The model under review builds one solid part; all positions refer to its coordinate system, in mm. Face numbers are marked on the shaded views. A direction names the side the tool comes from. Round coordinates to 2 decimals unless told otherwise and drop trailing zeros. Loops run counter-clockwise (first coordinate to the right, second up) from the corner with the lowest first, then second, coordinate; pieces in that order, holes last. Notation, with made-up numbers: (86, -11) -> (140, -11) arc R9 cw to (140, 2) -> close; hole circle Ø11 at (3, 86). An arc over 180 degrees is marked (long way). Use a Markdown table: item, result. Add a question column.
1) Insertion check: pin 1 (2 mm diameter, centred on y = -3.5, z = 5, fed in from +X); pin 2 (1.5 mm diameter, centred on x = 0.5, z = 12, fed in from -Y); pin 3 (2.5 mm diameter, centred on x = 0.5, y = 0, fed in from -Z). Each pin has a flat end and moves straight along its axis. Give the tip position at first contact, or say it passes through.
2) Wall thickness on probe 1 along Y at (x, z) = (0, 44); probe 2 along Z at (x, y) = (0.25, 3.25); probe 3 along Z at (x, y) = (-1.75, 0.5): over which ranges is each line inside the solid? List them lowest first.
3) For the marked faces 1 and 2, list the 3-axis set-ups (+Z, -Z, +X, -X, +Y, -Y) from which the entire face can be reached by the end or side of a thin tool; tool diameter is ignored.
4) Consider section A-A on y = 0. Give the boundary of the cut face in (x, z).
5) Consider section B-B on z = 41.5. Give the boundary of the cut face in (x, y).
from build123d import *

# Parameters (mm, degrees)
F0_R     = 4.73075
F1_DEPTH = 6.35
F2_R     = 3.0988
F3_DEPTH = 40.64
F5_DEPTH = 4.318
F6_SIZE  = 0.508


with BuildPart() as f1:
    # F0 (on Top) → F1 (new body)
    with BuildSketch(Plane.XY):
        Circle(F0_R)
    extrude(amount=F1_DEPTH)

    # F2 (on face) → F3 (join)
    with BuildSketch(Plane.XY.offset(6.35)):
        Circle(F2_R)
    extrude(amount=F3_DEPTH)

    # F4 (on face) → F5 (cut)
    with BuildSketch(Plane(origin=(0, 0, 0), x_dir=(1, 0, 0), z_dir=(0, 0, -1))):
        Polygon((2.38125, -1.374815), (2.38125, 1.374815), (0, 2.749631), (-2.38125, 1.374815), (-2.38125, -1.374815), (0, -2.749631), align=None)
    extrude(amount=-F5_DEPTH, mode=Mode.SUBTRACT)

    # F6
    f6_edges = [f1.edges().sort_by_distance(p)[0] for p in [
        (1.190625, 2.062223, 0),
        (2.38125, 0, 0),
        (1.190625, -2.062223, 0),
        (-1.190625, -2.062223, 0),
        (-2.38125, 0, 0),
        (-1.190625, 2.062223, 0),
        (-4.73075, 0, 0),
        (-4.73075, 0, 6.35),
        (-3.0988, 0, 46.99),
    ]]
    chamfer(f6_edges, length=F6_SIZE)


solid = f1.part
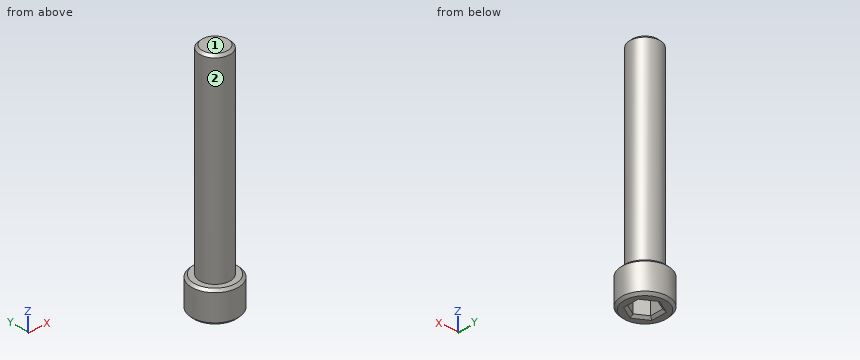
Result set:
| question | item | result |
|---|---|---|
| 1 | pin 1 | x = 4.02 |
| 1 | pin 2 | y = -3.1 |
| 1 | pin 3 | z = 4.32 |
| 2 | probe 1 | -3.1 to 3.1 |
| 2 | probe 2 | 0 to 6.35 |
| 2 | probe 3 | 4.32 to 46.99 |
| 3 | face 1 | +Z, +X, -X, +Y, -Y |
| 3 | face 2 | +Z |
| 4 | outline | (-4.73, 0.51) -> (-4.22, 0) -> (-2.89, 0) -> (-2.38, 0.51) -> (-2.38, 4.32) -> (2.38, 4.32) -> (2.38, 0.51) -> (2.89, 0) -> (4.22, 0) -> (4.73, 0.51) -> (4.73, 5.84) -> (4.22, 6.35) -> (3.1, 6.35) -> (3.1, 46.48) -> (2.59, 46.99) -> (-2.59, 46.99) -> (-3.1, 46.48) -> (-3.1, 6.35) -> (-4.22, 6.35) -> (-4.73, 5.84) -> close |
| 5 | outline | circle Ø6.2 at (0, 0) |
